Autodesk Inventor part; units mm, degrees
ref_plane "YZ Plane" through (0, 0, 0) normal (1, 0, 0) x (0, 1, 0)
ref_plane "XZ Plane" through (0, 0, 0) normal (0, 1, 0) x (-1, 0, 0)
ref_plane "XY Plane" through (0, 0, 0) normal (0, 0, 1) x (1, 0, 0)
sketch "Эскиз1" plane through (0, 0, 0) normal (0, 0, 1) x (1, 0, 0)
  circle A0 centre (0, 0) radius 1.5
  dimension "d0" = 3
extrude "Выдавливание1" add sketch "Эскиз1" along normal blind 20.25
sketch "Эскиз2" plane through (0, 0, 20.25) normal (0, 0, 1) x (1, 0, 0)
  line L0 (-1.5, -1) -> (1.5, -1)
  line L1 (1.5, -1) -> (1.5, 1)
  line L2 (1.5, 1) -> (-1.5, 1)
  line L3 (-1.5, 1) -> (-1.5, -1)
  line L4 (-1.5, -1) -> (1.5, 1) construction
  line L5 (1.5, -1) -> (-1.5, 1) construction
  circle A0 centre (0, 0) radius 1.5
  point P0 (-1.118, 1)
  point P1 (1.118, 1)
  dimension "d3" = 2
extrude "Выдавливание2" cut sketch "Эскиз2" against normal blind 3 contours A0 L2
sketch "Эскиз3" plane through (0, 0, 0) normal (0, 0, -1) x (-1, 0, 0)
  arc A0 (1.118, 1) -> (-1.118, 1) centre (0, 0) ccw
  line L0 (-1.118, 1) -> (1.118, 1)
extrude "Выдавливание3" cut sketch "Эскиз3" against normal blind 5
equation "\"Радиус_гибки\" = Толщина"
equation "\"Ширина_просечки\" = Толщина"
equation "\"Глубина_просечки\" = 0.5 * Толщина"
equation "\"Размер_просечки\" = 4 * Толщина"
equation "\"Мин_остаток\" = 2 * Толщина"
equation "\"Радиус_перехода\" = Радиус_гибки"
equation "\"Радиус_Якоби\" = Толщина"
equation "\"Размер_зазора\" = Толщина"
properties part number "Ось 3мм задняя"
Geometry check sheet. Reference: the model listing, model coordinates, mm. A direction names the side the tool comes from. Coordinates: 2 decimals unless noted, no trailing zeros. Loops run counter-clockwise (first coordinate to the right, second up) from the corner with the lowest first, then second, coordinate; pieces in that order, holes last. Notation, with made-up numbers: (71, -6) - (97, -6) arc R19 ccw to (97, 30) - close; hole circle Ø6 at (34, 35). An arc over 180 degrees is marked (long way). Use one line per item in the form item = value. Start each with the question number.
Item 1: Gauge pin test, flat ends, axial feed: pin 1 (0.7 mm diameter, centred on x = 0, z = 3.5, fed in from +Y); pin 2 (1 mm diameter, centred on y = -0.5, z = 16, fed in from -X). Record the tip position at first contact, or that the pin passes through.
Item 2: Mould release check, pull along Y, two halves, no side actions. Record for faces 1 (the face through (-0.195, -1.487, 9.983)), 2 (the face through (0, 0, 20.25)), 3 (the face through (0, 1, 2)): +Y half, -Y half, draft (parallel to the pull), parting line (faces both ways), or undercut.
Item 3: Section check D-D, the plane z = 6. Enter the section's corners in (x, y), and give its area (3 significant figures).
Item 4: Section check B-B, the plane z = 18.75. Enter the section's corners in (x, y).
Item 5: Section check C-C, the plane y = 0.6. Enter the section's corners in (x, z), and give its area (3 significant figures).
Item 6: Section check A-A, the plane x = 0. Enter the section's corners in (y, z).
Item 7: Thickness scan on probe 1 along X at (y, z) = (1, 8.25); probe 2 along X at (y, z) = (0.95, 5.5); probe 3 along Y at (x, z) = (-0.3, 6.25). Record the ranges inside material, lowest first.
Item 8: Tool access check on faces 4 (the face through (0, 1, 19)), 5 (the face through (0, 0, 0)). Record the directions out of +Z, -Z, +X, -X, +Y, -Y that give a thin tool (end or side, any length) a straight path to the whole face; none if there is none.
Computed:
q1.pin_1 = 1
q1.pin_2 = -1.5
q2.face_1 = parting line
q2.face_2 = draft
q2.face_3 = +Y half
q3.outline = circle Ø3 at (0, 0)
q3.area = 7.07 mm2
q4.outline = (-1.12, 1) arc R1.5 ccw (long way) to (1.12, 1) - close
q5.outline = (-1.37, 0) - (1.37, 0) - (1.37, 20.25) - (-1.37, 20.25) - close
q5.area = 55.7 mm2
q6.outline = (-1.5, 0) - (1, 0) - (1, 5) - (1.5, 5) - (1.5, 17.25) - (1, 17.25) - (1, 20.25) - (-1.5, 20.25) - close
q7.probe_1 = -1.12 to 1.12
q7.probe_2 = -1.16 to 1.16
q7.probe_3 = -1.47 to 1.47
q8.face_4 = +Z, +X, -X, +Y
q8.face_5 = -Z, +X, -X, +Y, -Y
